```python
from build123d import *

# Parameters (mm, degrees)
BOSS_EXTRUDE1_DEPTH      = 60
BOSS_EXTRUDE1_DEPTH_BACK = 20


with BuildPart() as part:
    # Sketch1 → Boss-Extrude1 (new, two sides: drawn at the far end of the back side and taken through both)
    with BuildSketch(Plane(origin=(190.645148, 0, 0), x_dir=(0, 0, -1), z_dir=(1, 0, 0)).offset(-BOSS_EXTRUDE1_DEPTH_BACK)):
        with BuildLine():
            Line((-246.970904961, 208.163538159), (-246.970904961, 205.163538159))
            Line((-246.970904961, 205.163538159), (-246.970904961, 197.163538159))
            Line((-246.970904961, 197.163538159), (-246.970904961, 194.163538159))
            Line((-246.970904961, 194.163538159), (-240.970904961, 194.163538159))
            Line((-240.970904961, 194.163538159), (-240.970904961, 197.163538159))
            Line((-240.970904961, 197.163538159), (-240.970904961, 199.913538158))
            Line((-240.970904961, 199.913538158), (-241.570904961, 199.913538158))
            ThreePointArc((-241.570904961, 199.913538158), (-242.820904961, 201.163538162), (-241.570904955, 202.413538158))
            Line((-241.570904955, 202.413538158), (-240.970904961, 202.413538158))
            Line((-240.970904961, 202.413538158), (-240.970904961, 205.163538159))
            Line((-240.970904961, 205.163538159), (-240.970904961, 208.163538159))
            Line((-240.970904961, 208.163538159), (-246.970904961, 208.163538159))
        make_face()
    extrude(amount=BOSS_EXTRUDE1_DEPTH + BOSS_EXTRUDE1_DEPTH_BACK)


solid = part.part
```
Could you check a few things on this model? Use its own coordinates, in mm. Coordinates: 2 decimals unless noted, no trailing zeros. Write each loop counter-clockwise with the first axis right and the second up, starting at its lowest first coordinate (ties: lowest second). Pieces come first, ordered by that corner, then holes. Notation, with made-up numbers: (0.25, 7.5) -> (59.25, 7.5) arc R26 cw to (59.25, 42.5) -> close; hole circle Ø7 at (-26.75, -37). An arc over 180 degrees is marked (long way). Return JSON: item names as keys, results as strings.
(1) We'd pull the mould along Y, two halves only. Please class faces 1 (the cylindrical face through (210.09, 201.14, 242.82)), 2 (the flat face through (210, 194.164, 244)), 3 (the flat face through (170.645, 201, 244)), 4 (the flat face through (210, 208.164, 244)): +Y half, -Y half, draft (parallel to the pull), parting line (faces both ways), or undercut.
Numbers:
{"face 1": "undercut", "face 2": "-Y half", "face 3": "draft", "face 4": "+Y half"}
(2) Imagine slicing it at B-B, the plane y = 200.75. Please give me the cut outline in (x, z).
Numbers:
{"outline": "(170.65, 242.75) -> (250.65, 242.75) -> (250.65, 246.97) -> (170.65, 246.97) -> close"}
(3) I need wall thicknesses on L1, parallel to Y at x = 236.5, z = 241.5; L2, parallel to Y at x = 236.5, z = 242.2; L3, parallel to Z at x = 188, y = 202. Which ranges of each line are inside material? Lowest first, please.
Numbers:
{"L1": "y = 194.16 to 199.91, 202.41 to 208.16", "L2": "y = 194.16 to 200.08, 202.24 to 208.16", "L3": "z = 242.5 to 246.97"}
(4) Imagine slicing it at A-A, the plane x = 233. Please give me the cut outline in (y, z).
Numbers:
{"outline": "(194.16, 240.97) -> (199.91, 240.97) -> (199.91, 241.57) arc R1.25 cw to (202.41, 241.57) -> (202.41, 240.97) -> (208.16, 240.97) -> (208.16, 246.97) -> (194.16, 246.97) -> close"}
